Work out the finished part from the listing and answer in its coordinate system (mm). Face numbers are marked on the shaded views. Coordinates: 2 decimals unless noted, no trailing zeros. Order: outer loops, then holes, each group sorted by start corner. A loop starts at its lowest first (then second) coordinate and runs counter-clockwise, first axis right, second up. Notation, with made-up numbers: M -26,79.25 L 0,79.25 A16 cw 0,97.25 Z; hole C -14,85 d6. An arc over 180 degrees is marked long. Use a Markdown table: item, result.
from build123d import *

# Parameters (mm, degrees)
F0_R      = 35.0672788862
F1_DEPTH  = 63.5
F2_R      = 11.0181598278
F3_DEPTH  = 12.7
F4_R      = 6.6894153835
F5_DEPTH  = 69.85
F7_START  = 50.8
F7_DEPTH  = 19.05
F9_START  = 6.35
F8_R      = 11.0281331537
F9_DEPTH  = 12.7
F11_START = 6.35
F10_R     = 11.0120586673
F11_DEPTH = 12.7
F13_START = 6.35
F12_R     = 11.0736476733
F13_DEPTH = 12.7
F18_R     = 23.0898876608
F19_DEPTH = 63.5


with BuildPart() as f1:
    # F0 (on Front) → F1 (new body)
    with BuildSketch(Plane.XZ):
        Circle(F0_R)
    extrude(amount=-F1_DEPTH)

    # F2 (on face) → F3 (join)
    with BuildSketch(Plane.XZ):
        Circle(F2_R)
    extrude(amount=F3_DEPTH)

    # F4 (on face) → F5 (join)
    with BuildSketch(Plane.XZ.offset(12.7)):
        Circle(F4_R)
    extrude(amount=F5_DEPTH)

    # F6 (on face) → F7 (join)
    with BuildSketch(Plane.XZ.offset(12.7).offset(F7_START)):
        Polygon((-5.5090799139, -9.5420063138), (5.5090799139, -9.5420063138), (11.0181598278, 0), (5.5090799139, 9.5420063138), (-5.5090799139, 9.5420063138), (-11.0181598278, 0), align=None)
    extrude(amount=F7_DEPTH)

    # F8 (on face) → F9 (join)
    with BuildSketch(Plane.XZ.offset(12.7).offset(F9_START)):
        Circle(F8_R)
    extrude(amount=F9_DEPTH)

    # F10 (on face) → F11 (join)
    with BuildSketch(Plane.XZ.offset(31.75).offset(F11_START)):
        Circle(F10_R)
    extrude(amount=F11_DEPTH)

    # F12 (on face) → F13 (join)
    with BuildSketch(Plane.XZ.offset(50.8).offset(F13_START)):
        Circle(F12_R)
    extrude(amount=F13_DEPTH)

    # F14 (on face) → F15 (revolve, cut)
    with BuildSketch(Plane(origin=(0, 63.5, 0), x_dir=(-1, 0, 0), z_dir=(0, 1, 0))):
        with BuildLine():
            ThreePointArc((-34.6572299507, -5.3470048278), (0, -35.0672788862), (34.6572299507, -5.3470048278))
            Line((34.6572299507, -5.3470048278), (18.4994737599, -5.3470048278))
            Line((18.4994737599, -5.3470048278), (-18.4994737599, -5.3470048278))
            Line((-18.4994737599, -5.3470048278), (-34.6572299507, -5.3470048278))
        make_face()
    revolve(axis=Axis((-2.320465399, 63.5, -46.4284271002), (-1, 0, 0)), mode=Mode.SUBTRACT)

    # F16 (on face) → F17 (revolve, cut)
    with BuildSketch(Plane(origin=(0, 63.5, 0), x_dir=(-1, 0, 0), z_dir=(0, 1, 0))):
        with BuildLine():
            ThreePointArc((34.3176019657, 7.2122287682), (0, 40.5588116187), (-34.3176019657, 7.2122287682))
            Line((-34.3176019657, 7.2122287682), (34.3176019657, 7.2122287682))
        make_face()
    revolve(axis=Axis((-9.9174939096, 63.5, 48.9058308303), (-1, 0, 0)), mode=Mode.SUBTRACT)

    # F18 (on Top) → F19 (cut, symmetric)
    with BuildSketch(Plane.XY):
        with Locations((0, 63.5572820902)):
            Circle(F18_R)
    extrude(amount=F19_DEPTH, both=True, mode=Mode.SUBTRACT)


solid = f1.part
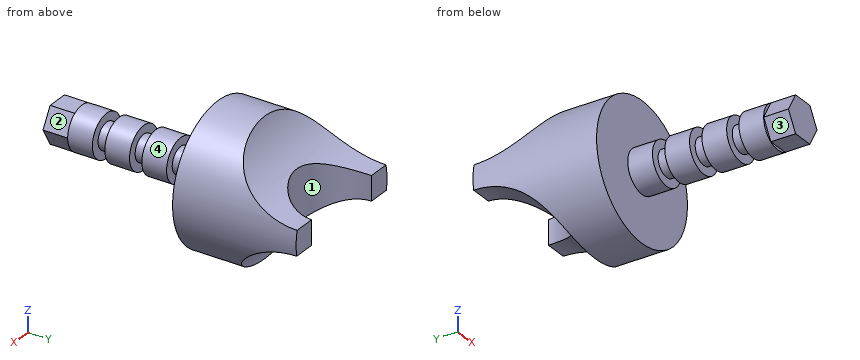
1. For a pull along X with two mould halves and no side action, classify the marked faces 1, 2, 3 and 4 as +X half, -X half, draft (parallel to the pull), parting line (faces both ways), or undercut.
Answers below:
| item | result |
|---|---|
| face 1 | undercut |
| face 2 | +X half |
| face 3 | -X half |
| face 4 | parting line |
2. Section A-A on y = -61.5 is taken. Determine the outline of the cut face in (x, z), then the cut area to 3 significant figures.
Answers below:
| item | result |
|---|---|
| outline | C 0,0 d22.15 |
| area | 385 mm² |
3. Section D-D on y = -23.5 is taken. Determine the outline of the cut face in (x, z).
Answers below:
| item | result |
|---|---|
| outline | C 0,0 d22.06 |
4. Flat-ended cylindrical pins translate along their axes: P1, Ø24.5, axis at x = -4.5, z = -2, coming from the +Y side; P2, Ø12, axis at x = -11, z = -16, coming from the -Y side; P3, Ø24.5, axis at x = 3, z = -0.5, coming from the +Y side; P4, Ø12, axis at x = -20, y = -63, coming from the -Z side. Find the tip coordinate at first contact, or state that the pin passes through.
Answers below:
| item | result |
|---|---|
| P1 | y = 47.66 |
| P2 | y = 0 |
| P3 | y = 46.22 |
| P4 | through |
5. Find the intervals of material crossed by probe 1 along Y at (x, z) = (-31, -2.5); probe 2 along Z at (x, y) = (1.5, 14.5); probe 3 along Y at (x, z) = (-12, 10), in increasing order.
Answers below:
| item | result |
|---|---|
| probe 1 | 0 to 63.5 |
| probe 2 | -35.04 to 35.04 |
| probe 3 | 0 to 43.83 |
6. Section B-B on x = -26 is taken. Determine the outline of the cut face in (y, z).
Answers below:
| item | result |
|---|---|
| outline | M 0,-23.53 L 29.39,-23.53 A41.08 cw 63.5,-5.35 L 63.5,7.21 A41.69 cw 30.42,23.53 L 0,23.53 Z |
7. Section C-C on x = 29 is taken. Determine the outline of the cut face in (y, z).
Answers below:
| item | result |
|---|---|
| outline | M 0,-19.72 L 32.29,-19.72 A41.08 cw 63.5,-5.35 L 63.5,7.21 A41.69 cw 33.73,19.72 L 0,19.72 Z |
